from build123d import *

# Parameters (mm, degrees)
F1_DEPTH = 63.5
F2_DEPTH = 7.9375
F3_DEPTH = 25.4
F4_DEPTH = 30.226


with BuildPart() as f1:
    # F0 (on Front) → F1 (new body, symmetric)
    with BuildSketch(Plane.XZ):
        Polygon((-41.275, 9.525), (-41.275, -9.525), (41.275, -9.525), (41.275, 9.525), (22.225, 9.525), align=None)
    extrude(amount=F1_DEPTH, both=True)

    # F0 (on Front) → F2 (join, symmetric)
    with BuildSketch(Plane.XZ):
        with BuildLine():
            add(Edge.make_bspline(
                [(-41.275, 9.525), (-29.9963708967, 51.1887520552), (24.8447079211, 65.5416920781), (57.15, 61.9252)],
                knots=[0, 0, 0, 0, 111.5045361635, 111.5045361635, 111.5045361635, 111.5045361635], degree=3))
            Line((-41.275, 9.525), (22.225, 9.525))
            Line((22.225, 9.525), (22.225, 27.0002))
            ThreePointArc((22.225, 27.0002), (32.4542956671, 51.6959043329), (57.15, 61.9252))
        make_face()
    extrude(amount=F2_DEPTH, both=True)

    # F0 (on Front) → F3 (join, symmetric)
    with BuildSketch(Plane.XZ):
        with BuildLine():
            Line((22.225, 9.525), (41.275, 9.525))
            Line((41.275, 9.525), (41.275, 27.0002))
            ThreePointArc((41.275, 27.0002), (45.9246798487, 38.2255201513), (57.15, 42.8752))
            Line((57.15, 42.8752), (60.325, 42.8752))
            Line((60.325, 42.8752), (60.325, 61.9252))
            Line((60.325, 61.9252), (57.15, 61.9252))
            ThreePointArc((57.15, 61.9252), (32.4542956671, 51.6959043329), (22.225, 27.0002))
            Line((22.225, 27.0002), (22.225, 9.525))
        make_face()
    extrude(amount=F3_DEPTH, both=True)

    # F0 (on Front) → F4 (join, symmetric)
    with BuildSketch(Plane.XZ):
        Polygon((85.6958447059, 42.8752), (60.325, 42.8752), (60.325, 38.1), (85.725, 38.1), align=None)
        Polygon((60.325, 66.675), (60.325, 61.9252), (85.5795336922, 61.9252), (85.5505334795, 66.675), align=None)
        Polygon((85.5795336922, 61.9252), (60.325, 61.9252), (60.325, 42.8752), (85.6958447059, 42.8752), align=None)
        Polygon((85.5505334795, 66.675), (85.5795336922, 61.9252), (85.6267288327, 61.9252), (85.7430398464, 42.8752), (85.6958447059, 42.8752), (85.725, 38.1), (111.125, 38.1), (111.125, 66.675), align=None)
    extrude(amount=F4_DEPTH, both=True)


solid = f1.part
Geometry: final body of the model. Coordinates: model frame, mm. A direction names the side the tool comes from. Round coordinates to 2 decimals unless told otherwise and drop trailing zeros. Write each loop counter-clockwise with the first axis right and the second up, starting at its lowest first coordinate (ties: lowest second). Pieces come first, ordered by that corner, then holes. Notation, with made-up numbers: M 44,-21 L 83,-21 A27 ccw 83,-3 Z; hole C 51.25,86 d1. An arc over 180 degrees is marked long. Write item = value, one per line.
Item 1: Section query C-C on y = -56. Return loops of the section in (x, z) (3 decimals).
Findings:
outline = M -41.275,-9.525 L 41.275,-9.525 L 41.275,9.525 L -41.275,9.525 Z
Item 2: Pull-direction query (X, two-part tool) for faces 5 (the face through (37, -25.4, 36)), 6 (the face through (32.73, -16.79, 51.97)), 7 (the face through (60.325, -0.4, 62.1)), 8 (the face through (41.275, -1, 4)); classes: pulls with the +X half, pulls with the -X half, needs draft (parallel to the pull), parting line crosses it, or undercut.
Findings:
face_5 = needs draft
face_6 = pulls with the -X half
face_7 = undercut
face_8 = pulls with the +X half
Item 3: Access query for faces 1 (the face through (22.225, 17, 18)), 2 (the face through (-41.275, -1, 0)), 3 (the face through (85, 0, 38.1)), 4 (the face through (-2, -7.938, 32)). Directions: +Z, -Z, +X, -X, +Y, -Y. A direction counts if a zero-diameter tool reaches every point of the face in a straight line with its end or side. Return the directions, or none.
Findings:
face_1 = +Z, -X, +Y
face_2 = +Z, -Z, -X, +Y, -Y
face_3 = -Z, +X, +Y, -Y
face_4 = +Z, -X, -Y
Item 4: Section query B-B on x = 78. Return loops of the section in (y, z) (3 decimals).
Findings:
outline = M -30.226,38.1 L 30.226,38.1 L 30.226,66.675 L -30.226,66.675 Z
Item 5: Material intervals for line 1 along Z through (x, y) = (-29.5, 41) (3 decimals); line 2 along X through (y, z) = (53, 0) (3 decimals); line 3 along X through (y, z) = (-17.5, 16.5) (3 decimals), sorted ascending. Write a range as [from, to].
Findings:
line_1 = [-9.525, 9.525]
line_2 = [-41.275, 41.275]
line_3 = [22.225, 41.275]
Item 6: Pin query (flat end, axial travel): P1, Ø15, axis at x = 77, y = 3, coming from the -Z side; P2, Ø8.5, axis at y = -20.5, z = 21.5, coming from the -X side (3 decimals); P3, Ø19, axis at y = 13, z = 14.5, coming from the -X side (3 decimals); P4, Ø5, axis at y = 48, z = -1, coming from the +X side (3 decimals). Return the tip coordinate at first contact, or that it passes through.
Findings:
P1 = 38.1
P2 = 22.225
P3 = -41.275
P4 = 41.275
Item 7: Section query A-A on y = 14. Return loops of the section in (x, z) (3 decimals), then the cut area to 3 significant figures.
Findings:
outline = M -41.275,-9.525 L 41.275,-9.525 L 41.275,27 A15.875 cw 57.15,42.875 L 60.325,42.875 L 60.325,38.1 L 111.125,38.1 L 111.125,66.675 L 60.325,66.675 L 60.325,61.925 L 57.15,61.925 A34.925 ccw 22.225,27 L 22.225,9.525 L -41.275,9.525 Z; hole M 85.58,61.925 L 85.696,42.875 L 85.743,42.875 L 85.627,61.925 Z
area = 4,180 mm^2
